Autodesk Inventor part; units mm, degrees
ref_plane "YZ Plane" through (0, 0, 0) normal (1, 0, 0) x (0, 1, 0)
ref_plane "XZ Plane" through (0, 0, 0) normal (0, 1, 0) x (-1, 0, 0)
ref_plane "XY Plane" through (0, 0, 0) normal (0, 0, 1) x (1, 0, 0)
sketch "Sketch1" plane through (0, 0, 0) normal (0, 0, 1) x (1, 0, 0)
  line L0 (-3, 3) -> (3, 3)
  line L1 (3, 3) -> (3, -3)
  line L2 (3, -3) -> (-3, -3)
  line L3 (-3, -3) -> (-3, 3)
  line L4 (-3, 3) -> (3, -3) construction
  line L5 (3, 3) -> (-3, -3) construction
  line L6 (0, 1) -> (3, 1)
  line L7 (3, 1) -> (3, -1)
  line L8 (3, -1) -> (0, -1)
  line L9 (0, -1) -> (0, 1)
  line L10 (0, 1) -> (3, -1) construction
  line L11 (3, 1) -> (0, -1) construction
  line L12 (0, 1) -> (0, 2)
  line L13 (0, 2) -> (1.5, 0)
  line L14 (0, -1) -> (0, -2)
  line L15 (0, -2) -> (1.5, 0)
  point P0 (0, 0)
  point P1 (0.75, -1)
  point P2 (0.75, 1)
  dimension "d0" = 6
  dimension "d1" = 2
  dimension "d2" = 3
  dimension "d3" = 1
extrude "Extrusion1" add sketch "Sketch1" along normal blind 200 contours L0 L1 L6 L13 L12 L9 L14 L15 L8 L2 L3
chamfer "Chamfer1" distance 1 angle 45 2 edges at (3, 1, 100) (3, -1, 100)
properties part number "LinearRail"
Geometry: final body of the model. Coordinates: model frame, mm. Round coordinates to 2 decimals unless told otherwise and drop trailing zeros. Order: outer loops, then holes, each group sorted by start corner. A loop starts at its lowest first (then second) coordinate and runs counter-clockwise, first axis right, second up. Notation, with made-up numbers: (41, 66) -> (55, 66) arc R19 ccw to (55, 103) -> close; hole circle Ø11 at (22, 72.5). An arc over 180 degrees is marked (long way). Use CSV: the item, a comma, the result in double quotes. Start each with the question number.
1) Material intervals for line 1 along Y through (x, z) = (1.75, 88.5); line 2 along X through (y, z) = (-0.9, 73); line 3 along X through (y, z) = (1.15, 70.5), sorted ascending. Write a range as from..to.
2) Draft query along X for faces 1 (the face through (-1, 0, 200)), 2 (the face through (0, 0, 99)), 3 (the face through (-3, 0, 99)). Return one class per face: +X half, -X half, draft (parallel to the pull), parting line (faces both ways), or undercut.
3) Section A-A (z = 77). Return the cut outline in (x, y).
4) First-contact query: pin 1 Ø1.2 at (y, z) = (-1, 88) entering from +X. Flat tip, straight axial feed; report the tip coordinate or a pass-through.
Returned:
1,line 1,"y = -3..-1, 1..3"
1,line 2,"x = -3..0"
1,line 3,"x = -3..0, 0.64..2.15"
2,face 1,"draft"
2,face 2,"undercut"
2,face 3,"-X half"
3,outline,"(-3, -3) -> (3, -3) -> (3, -2) -> (2, -1) -> (0.75, -1) -> (0, -2) -> (0, 2) -> (0.75, 1) -> (2, 1) -> (3, 2) -> (3, 3) -> (-3, 3) -> close"
4,pin 1,"stops at x = 2.6"
